```python
from build123d import *

# Parameters (mm, degrees)
F0_R      = 6
F1_DEPTH  = 3
F2_R      = 4.8
F3_DEPTH  = 1.15
F4_R      = 6
F4_R_2    = 4.8
F5_DEPTH  = 20
F6_R      = 8
F6_R_2    = 6
F7_DEPTH  = 665
F8_R      = 6
F9_DEPTH  = 20
F10_R     = 4.8
F11_DEPTH = 1.15
F12_R     = 6
F12_R_2   = 4.8
F13_DEPTH = 3
F14_R     = 5
F15_DEPTH = 15
F16_SIZE  = 1


with BuildPart() as f1:
    # F0 (on Top) → F1 (new body)
    with BuildSketch(Plane.XY):
        Circle(F0_R)
    extrude(amount=F1_DEPTH)

    # F2 (on face) → F3 (join)
    with BuildSketch(Plane.XY.offset(3)):
        Circle(F2_R)
    extrude(amount=F3_DEPTH)

    # F4 (on face) → F5 (join)
    with BuildSketch(Plane.XY.offset(4.15)):
        Circle(F4_R)
        Circle(F4_R_2, mode=Mode.SUBTRACT)
        Circle(F4_R_2)
    extrude(amount=F5_DEPTH)

    # F6 (on face) → F7 (join)
    with BuildSketch(Plane.XY.offset(24.15)):
        Circle(F6_R)
        Circle(F6_R_2, mode=Mode.SUBTRACT)
        Circle(F6_R_2)
    extrude(amount=F7_DEPTH)

    # F8 (on face) → F9 (join)
    with BuildSketch(Plane.XY.offset(689.15)):
        Circle(F8_R)
    extrude(amount=F9_DEPTH)

    # F10 (on face) → F11 (join)
    with BuildSketch(Plane.XY.offset(709.15)):
        Circle(F10_R)
    extrude(amount=F11_DEPTH)

    # F12 (on face) → F13 (join)
    with BuildSketch(Plane.XY.offset(710.3)):
        Circle(F12_R)
        Circle(F12_R_2, mode=Mode.SUBTRACT)
        Circle(F12_R_2)
    extrude(amount=F13_DEPTH)

    # F14 (on face) → F15 (join)
    with BuildSketch(Plane.XY.offset(713.3)):
        Circle(F14_R)
    extrude(amount=F15_DEPTH)

    # F16
    f16_edges = [f1.edges().sort_by_distance(p)[0] for p in [
        (-5, 0, 728.3),
        (-6, 0, 0),
    ]]
    chamfer(f16_edges, length=F16_SIZE)


solid = f1.part
```
Read the model definition and answer for the solid it produces. Units are mm, in the model's axes. A direction names the side the tool comes from. Round coordinates to 2 decimals unless told otherwise and drop trailing zeros. Write each loop counter-clockwise with the first axis right and the second up, starting at its lowest first coordinate (ties: lowest second). Pieces come first, ordered by that corner, then holes. Notation, with made-up numbers: (-17, -22) - (18, -22) arc R28 cw to (18, 7) - close; hole circle Ø11 at (4.5, 5.25). An arc over 180 degrees is marked (long way). One line per item, written item: value.
Q1. For a pull along Z with two mould halves and no side action, classify faces 4 (the cylindrical face through (-1.73, -7.81, 351.99)), 5 (the flat face through (-2, 6, 689.15)), 6 (the flat face through (-3, 4, 710.3)) as pulls with the +Z half, pulls with the -Z half, needs draft (parallel to the pull), parting line crosses it, or undercut.
The answers:
face 4: needs draft
face 5: pulls with the +Z half
face 6: undercut
Q2. Find section A-A (z = 196.5). Determine the outline of the cut face in (x, y).
The answers:
outline: circle Ø16 at (0, 0)
Q3. Straight lines are drawn through the part: line 1 (Z direction, x = -5.5, y = 2.25); line 2 (X direction, y = -5.25, z = 42); line 3 (Z direction, x = 1.25, y = 7). For each, find the intervals that lie inside material, in ascending order. Write a range as from..to.
The answers:
line 1: z = 0.94..3, 4.15..709.15, 710.3..713.3
line 2: x = -6.04..6.04
line 3: z = 24.15..689.15
Q4. Which of the six approach directions +Z, -Z, +X, -X, +Y, -Y give full straight-line access (tool end or side, diameter ignored) to faces 1 (the cylindrical face through (-6, 0, 14)), 2 (the cylindrical face through (-6, 0, 712)), 3 (the flat face through (-3, 4, 709.15))?
The answers:
face 1: -Z
face 2: +Z
face 3: none
Q5. Each of these flat-tipped pins is pushed along its axis until it touches: P1, Ø6, axis at x = 0, y = -3, coming from the -Z side; P2, Ø2, axis at x = -4.5, y = -5.5, coming from the -Z side; P3, Ø1, axis at x = 5.5, z = 510, coming from the -Y side (3 decimals); P4, Ø1.5, axis at y = -1, z = 434, coming from the -X side. Where does it stop, or does it pass through?
The answers:
P1: stops at z = 0
P2: stops at z = 24.15
P3: stops at y = -6.245
P4: stops at x = -8
